For this review, take the finished solid that the model builds, in its own axes (mm). Give positions to 0.01 mm unless a question says otherwise; leave off trailing zeros. Write each loop counter-clockwise with the first axis right and the second up, starting at its lowest first coordinate (ties: lowest second). Pieces come first, ordered by that corner, then holes. Notation, with made-up numbers: M 35.5,4 L 51.5,4 A7 cw 51.5,17 Z; hole C 86.25,6 d8. An arc over 180 degrees is marked long. Write item = value, one per line.
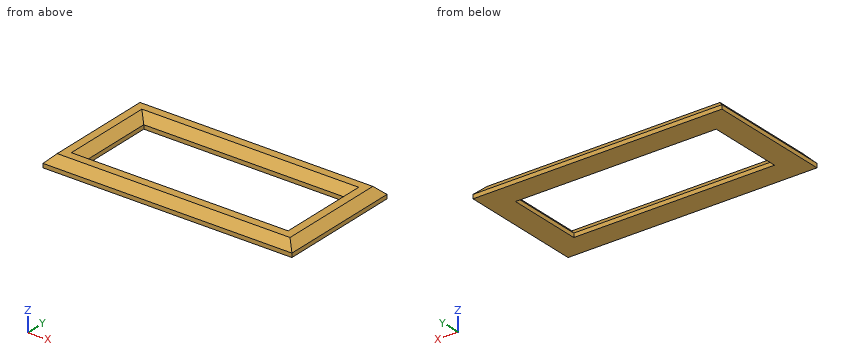
```python
from build123d import *

# Parameters (mm, degrees)
ESQUISSE1_W        = 62
ESQUISSE1_H        = 31
ESQUISSE1_W_2      = 50
ESQUISSE1_H_2      = 19
BOSS_EXTRU_1_DEPTH = 3
CHANFREIN1_SIZE    = 2


with BuildPart() as part:
    # Esquisse1 → Boss.-Extru.1 (new body)
    with BuildSketch(Plane.XY):
        with Locations((-25, 9.5)):
            Rectangle(ESQUISSE1_W, ESQUISSE1_H)
        with Locations((-25, 9.5)):
            Rectangle(ESQUISSE1_W_2, ESQUISSE1_H_2, mode=Mode.SUBTRACT)
    extrude(amount=BOSS_EXTRU_1_DEPTH)

    # Chanfrein1
    chanfrein1_edges = [part.edges().sort_by_distance(p)[0] for p in [
        (-56, 9.5, 3),
        (-25, -6, 3),
        (0, 9.5, 3),
        (-25, 19, 3),
        (-50, 9.5, 3),
        (-25, 0, 3),
        (6, 9.5, 3),
        (-25, 25, 3),
    ]]
    chamfer(chanfrein1_edges, length=CHANFREIN1_SIZE)


solid = part.part
```
1. Insertion check: P1, Ø1, axis at x = -24, z = 2.5, coming from the -Y side. The pin has a flat end and moves straight along its axis. Give the tip position at first contact, or say it passes through.
Responses:
P1 = -5
2. We need section B-B, the plane x = -4. Write out the cut boundary in (y, z).
Responses:
outline = M -6,0 L 0,0 L 0,1 L -2,3 L -4,3 L -6,1 Z; M 19,0 L 25,0 L 25,1 L 23,3 L 21,3 L 19,1 Z
3. We need section C-C, the plane z = 2.5. Write out the cut boundary in (x, y), then the cut area to 3 significant figures.
Responses:
outline = M -54.5,-4.5 L 4.5,-4.5 L 4.5,23.5 L -54.5,23.5 Z; hole M -51.5,-1.5 L 1.5,-1.5 L 1.5,20.5 L -51.5,20.5 Z
area = 486 mm2
4. We need section D-D, the plane x = -51. Write out the cut boundary in (y, z).
Responses:
outline = M -6,0 L 25,0 L 25,1 L 23,3 L 21,3 L 20,2 L -1,2 L -2,3 L -4,3 L -6,1 Z
5. We need section A-A, the plane y = 9.5. Write out the cut boundary in (x, z).
Responses:
outline = M -56,0 L -50,0 L -50,1 L -52,3 L -54,3 L -56,1 Z; M 0,0 L 6,0 L 6,1 L 4,3 L 2,3 L 0,1 Z
6. For line 1 along Y through (x, z) = (-48.5, 0.55); line 2 along X through (y, z) = (6, 0.2); line 3 along X through (y, z) = (-1, 2.2), list the stretches that pass through material, from the lowest coordinate up. Write a range as from..to.
Responses:
line_1 = -6..0, 19..25
line_2 = -56..-50, 0..6
line_3 = -54.8..-51.2, 1.2..4.8
